```python
from build123d import *

# Parameters (mm, degrees)
SKETCH1_R           = 24.5
SKETCH1_R_2         = 2.4999999999999996
SKETCH1_R_3         = 2.499999999999988
SKETCH1_R_4         = 2.5000000000000018
BOSS_EXTRUDE1_DEPTH = 10.530000000000001
SKETCH2_R           = 4
SKETCH2_R_2         = 2.4999999999999996
BOSS_EXTRUDE2_DEPTH = 14.5
SKETCH3_R           = 5
SKETCH3_R_2         = 4
BOSS_EXTRUDE3_DEPTH = 1.5
BOSS_EXTRUDE4_DEPTH = 14.5
FILLET2_R           = 0.5
FILLET5_R           = 1.5
CIRPATTERN1_START   = 10.53
CIRPATTERN1_DEPTH   = 14.5
SKETCH5_R           = 1.5000000000000442
CUT_EXTRUDE1_DEPTH  = 43.74343124745603
SKETCH6_R           = 2.7499999999999947
CUT_EXTRUDE2_DEPTH  = 3
SKETCH7_R           = 4.25
CUT_EXTRUDE3_DEPTH  = 5
CIRPATTERN2_COUNT   = 3
CHAMFER1_SIZE       = 0.5
SKETCH9_R           = 8
CUT_EXTRUDE4_DEPTH  = 38.559952245709795
BOSS_EXTRUDE7_START = -6.530000000000001
SKETCH10_R          = 8
SKETCH10_R_2        = 6.500000000000002
BOSS_EXTRUDE7_DEPTH = 6.530000000000001
CHAMFER2_SIZE       = 0.5
BOSS_EXTRUDE8_START = -1.5
SKETCH11_R          = 26.000000000000007
SKETCH11_R_2        = 24.5
BOSS_EXTRUDE8_DEPTH = 1.5


# Read off the part's stored shape, not the designer's step: CirPattern1
with BuildPart() as part:
    # Sketch1 → Boss-Extrude1 (new body)
    with BuildSketch(Plane.XY):
        Circle(SKETCH1_R)
        with Locations((0, 19.5)):
            Circle(SKETCH1_R_2, mode=Mode.SUBTRACT)
        with Locations((16.887495373796185, -9.750000000000636)):
            Circle(SKETCH1_R_3, mode=Mode.SUBTRACT)
        with Locations((-16.887495373797307, -9.750000000000002)):
            Circle(SKETCH1_R_4, mode=Mode.SUBTRACT)
    extrude(amount=BOSS_EXTRUDE1_DEPTH)

    # Sketch2 → Boss-Extrude2 (add)
    with BuildSketch(Plane.XY.offset(10.530000000000001)):
        with Locations(Location((0, 19.5, 0), (0, 0, 180))):
            Circle(SKETCH2_R)
        with Locations((0, 19.5)):
            Circle(SKETCH2_R_2, mode=Mode.SUBTRACT)
    extrude(amount=BOSS_EXTRUDE2_DEPTH)

    # Sketch3 → Boss-Extrude3 (add)
    with BuildSketch(Plane.XY.offset(10.530000000000001)):
        with Locations(Location((0, 19.5, 0), (0, 0, 90))):
            Circle(SKETCH3_R)
        with Locations(Location((0, 19.5, 0), (0, 0, 180))):
            Circle(SKETCH3_R_2, mode=Mode.SUBTRACT)
    extrude(amount=BOSS_EXTRUDE3_DEPTH)

    # Sketch4 → Boss-Extrude4 (add)
    with BuildSketch(Plane.XY.offset(10.530000000000001)):
        with BuildLine():
            ThreePointArc((-8.496322733983213, 7.75), (-12.968536294458422, 13.01408708204353), (-14.497844667397978, 19.750000000000004))
            ThreePointArc((-14.497844667397978, 19.75), (-21.21762239271878, 12.249999999999943), (-24.352924058441666, 2.6805017820872727))
            ThreePointArc((-24.352924058441673, 2.6805017820872727), (-17.754798167341832, 4.724038339879645), (-10.959858246321023, 3.48303132638066))
            ThreePointArc((-10.959858246321025, 3.483031326380663), (-9.959292143521058, 5.749999999999978), (-8.496322733983213, 7.750000000000001))
        make_face()
    extrude(amount=BOSS_EXTRUDE4_DEPTH)

    # Fillet2
    fillet2_edges = [part.edges().sort_by_distance(p)[0] for p in [
        (-9.2e-16, 14.5, 12.030000000000001),
    ]]
    fillet(fillet2_edges, radius=FILLET2_R)

    # Fillet5
    fillet5_edges = [part.edges().sort_by_distance(p)[0] for p in [
        (-14.49784466739798, 19.75, 17.78),
        (-24.35292405844167, 2.6805017820872727, 17.78),
        (-10.959858246321025, 3.4830313263806616, 17.78),
        (-8.496322733983215, 7.75, 17.78),
    ]]
    fillet(fillet5_edges, radius=FILLET5_R)

    # CirPattern1 outline → CirPattern1 (add)
    with BuildSketch(Plane.XY.offset(CIRPATTERN1_START)):
        with BuildLine():
            ThreePointArc((-1.069906346, -11.450122288), (-2.103251355, -11.738985499), (-2.679275225, -12.644214953))
            ThreePointArc((-2.679275225, -12.644214953), (-4.43366395, -17.176444835), (-7.58708663, -20.874405476))
            ThreePointArc((-7.58708663, -20.874405476), (-8.094453803, -22.326259468), (-7.057038992, -23.461632523))
            ThreePointArc((-7.057038992, -23.461632523), (0, -24.5), (7.057038992, -23.461632523))
            ThreePointArc((7.057038992, -23.461632523), (8.094453803, -22.326259468), (7.58708663, -20.874405476))
            ThreePointArc((7.58708663, -20.874405476), (4.43366395, -17.176444835), (2.679275225, -12.644214953))
            ThreePointArc((2.679275225, -12.644214953), (2.103251355, -11.738985499), (1.069906346, -11.450122288))
            ThreePointArc((1.069906346, -11.450122288), (0, -11.5), (-1.069906346, -11.450122288))
        make_face()
        with BuildLine():
            ThreePointArc((23.846889276, 5.619241219), (21.217622393, 12.25), (16.789850284, 17.842391304))
            ThreePointArc((16.789850284, 17.842391304), (15.28788097, 18.173132357), (14.284222116, 17.0078125))
            ThreePointArc((14.284222116, 17.0078125), (12.658405598, 12.42788803), (9.610573748, 8.642427885))
            ThreePointArc((9.610573748, 8.642427885), (9.11463398, 7.690961853), (9.381143605, 6.651627219))
            ThreePointArc((9.381143605, 6.651627219), (9.959292144, 5.75), (10.451049951, 4.798495069))
            ThreePointArc((10.451049951, 4.798495069), (11.217885334, 4.048023646), (12.289848972, 4.001787068))
            ThreePointArc((12.289848972, 4.001787068), (17.092069548, 4.748556804), (21.871308746, 3.866592976))
            ThreePointArc((21.871308746, 3.866592976), (23.382334773, 4.153127111), (23.846889276, 5.619241219))
        make_face()
    extrude(amount=CIRPATTERN1_DEPTH)

    # CirPattern1 2 outline → CirPattern1 2 (revolve)
    with BuildSketch(Plane(origin=(-16.887495374, -9.75, 0), x_dir=(1, 0, 0), z_dir=(0, -1, 0))):
        with BuildLine():
            Line((4, 25.03), (2.5, 25.03))
            Line((2.5, 25.03), (2.5, 10.53))
            Line((2.5, 10.53), (5, 10.53))
            Line((5, 10.53), (5, 11.53))
            ThreePointArc((5, 11.53), (4.853553391, 11.883553391), (4.5, 12.03))
            Line((4.5, 12.03), (4, 12.03))
            Line((4, 12.03), (4, 25.03))
        make_face()
    revolve(axis=Axis((-16.887495374, -9.75, 0), (0, 0, 1)))

    # CirPattern1 3 outline → CirPattern1 3 (revolve)
    with BuildSketch(Plane(origin=(16.887495374, -9.75, 0), x_dir=(1, 0, 0), z_dir=(0, -1, 0))):
        with BuildLine():
            Line((4, 25.03), (2.5, 25.03))
            Line((2.5, 25.03), (2.5, 10.53))
            Line((2.5, 10.53), (5, 10.53))
            Line((5, 10.53), (5, 11.53))
            ThreePointArc((5, 11.53), (4.853553391, 11.883553391), (4.5, 12.03))
            Line((4.5, 12.03), (4, 12.03))
            Line((4, 12.03), (4, 25.03))
        make_face()
    revolve(axis=Axis((16.887495374, -9.75, 0), (0, 0, 1)))

    # Sketch5 → Cut-Extrude1 (cut, through all)
    with BuildSketch(Plane.XY.offset(25.030000000000005)):
        with Locations((-17.753520777581024, 10.249999999999956)):
            Circle(SKETCH5_R)
    cut_extrude1 = extrude(amount=-CUT_EXTRUDE1_DEPTH, mode=Mode.SUBTRACT)

    # Sketch6 → Cut-Extrude2 (cut)
    with BuildSketch(Plane(origin=(0, 0, 0), x_dir=(-1, 0, 0), z_dir=(0, 0, -1))):
        with Locations((17.753520777581024, 10.249999999999956)):
            Circle(SKETCH6_R)
    cut_extrude2 = extrude(amount=-CUT_EXTRUDE2_DEPTH, mode=Mode.SUBTRACT)

    # Sketch7 → Cut-Extrude3 (cut)
    with BuildSketch(Plane(origin=(0, 0, 0), x_dir=(-1, 0, 0), z_dir=(0, 0, -1))):
        with Locations((0, 19.5)):
            Circle(SKETCH7_R)
    cut_extrude3 = extrude(amount=-CUT_EXTRUDE3_DEPTH, mode=Mode.SUBTRACT)

    # CirPattern2: Cut-Extrude1, Cut-Extrude2, Cut-Extrude3 ×3 about axis
    cirpattern2_axis = Axis((1.3e-16, -8.9e-16, 0), (0, 0, 1))
    add([cut_extrude1.rotate(cirpattern2_axis, i * 360 / CIRPATTERN2_COUNT) for i in range(1, CIRPATTERN2_COUNT)], mode=Mode.SUBTRACT)
    add([cut_extrude2.rotate(cirpattern2_axis, i * 360 / CIRPATTERN2_COUNT) for i in range(1, CIRPATTERN2_COUNT)], mode=Mode.SUBTRACT)
    add([cut_extrude3.rotate(cirpattern2_axis, i * 360 / CIRPATTERN2_COUNT) for i in range(1, CIRPATTERN2_COUNT)], mode=Mode.SUBTRACT)

    # Chamfer1
    chamfer1_edges = [part.edges().sort_by_distance(p)[0] for p in [
        (-24.5, 3e-15, 0),
    ]]
    chamfer(chamfer1_edges, length=CHAMFER1_SIZE)

    # Sketch9 → Cut-Extrude4 (cut, through all)
    with BuildSketch(Plane.XY.offset(10.530000000000001)):
        Circle(SKETCH9_R)
    extrude(amount=-CUT_EXTRUDE4_DEPTH, mode=Mode.SUBTRACT)

    # Sketch10 → Boss-Extrude7 (add)
    with BuildSketch(Plane(origin=(0, 0, 0), x_dir=(-1, 0, 0), z_dir=(0, 0, -1)).offset(BOSS_EXTRUDE7_START)):
        with Locations(Location((0, 0, 0), (0, 0, 180))):
            Circle(SKETCH10_R)
        Circle(SKETCH10_R_2, mode=Mode.SUBTRACT)
    extrude(amount=BOSS_EXTRUDE7_DEPTH)

    # Chamfer2
    chamfer2_edges = [part.edges().sort_by_distance(p)[0] for p in [
        (-8, 9.8e-16, 10.530000000000001),
    ]]
    chamfer(chamfer2_edges, length=CHAMFER2_SIZE)

    # Sketch11 → Boss-Extrude8 (add)
    with BuildSketch(Plane.XY.offset(10.530000000000001).offset(BOSS_EXTRUDE8_START)):
        Circle(SKETCH11_R)
        Circle(SKETCH11_R_2, mode=Mode.SUBTRACT)
    extrude(amount=BOSS_EXTRUDE8_DEPTH)


solid = part.part
```
Check sheet for the modelled part. Datum: model origin and axes. Units: mm. A direction names the side the tool comes from. Round coordinates to 2 decimals unless told otherwise and drop trailing zeros. Order: outer loops, then holes, each group sorted by start corner. A loop starts at its lowest first (then second) coordinate and runs counter-clockwise, first axis right, second up. Notation, with made-up numbers: (-15.75, 20.25) -> (7.25, 20.25) arc R17 ccw to (7.25, 43.25) -> close; hole circle Ø5 at (-14, 71). An arc over 180 degrees is marked (long way). One line per item, written item: value. Start each with the question number.
Q1. Set-up check for faces 4 (the face through (9.952, 5.763, 17.678)), 5 (the face through (-0.22, 14.505, 11.023)), 6 (the face through (16, -7, 5)): record each of +Z, -Z, +X, -X, +Y, -Y from which the full face is reachable in a straight line by a thin tool's end or side.
Q2. Mould release check, pull along X, two halves, no side actions. Record for faces 1 (the face through (13.17, 20.66, 4.71)), 2 (the face through (17, 12, 3)), 3 (the face through (-16.9, -12.4, 25.03)): pulls with the +X half, pulls with the -X half, needs draft (parallel to the pull), parting line crosses it, or undercut.
Q3. Thickness scan on line 1 (Y direction, x = 0, z = 7.65); line 2 (Y direction, x = 16, z = 20.5); line 3 (X direction, y = 10.5, z = 21.5). Record the ranges inside material, lowest first.
Q4. Cross-section at C-C (x = -18.5). Give the number of separate pieces and of enclosed holes in the cut face, and give its area (3 significant figures).
Q5. Cross-section at B-B (z = 4). Record the boundary of the cut face in (x, y), and give its area (3 significant figures).
Q6. Cross-section at A-A (y = 0). Record the boundary of the cut face in (x, z).
Q7. Gauge pin test, flat ends, axial feed: pin 1 Ø6 at (x, z) = (-9.5, 19.5) entering from +Y; pin 2 Ø3 at (x, y) = (-19.5, 18.5) entering from -Z; pin 3 Ø3 at (y, z) = (-13, 9.5) entering from -X; pin 4 Ø3 at (y, z) = (-3.5, 13.5) entering from -X. Record the tip position at first contact, or that the pin passes through.
Completed:
1. face 4: +Z, -Y
1. face 5: +Z
1. face 6: -Z
2. face 1: parting line crosses it
2. face 2: undercut
2. face 3: needs draft
3. line 1: y = -24.5 to -22, -19 to -8, 8 to 17, 22 to 24.5
3. line 2: y = -13.65 to -12.09, -7.41 to -5.85, 4.72 to 18.23
3. line 3: x = -22.14 to -19.23, -16.27 to -11.37, 11.37 to 16.27, 19.23 to 22.14
4. separate pieces: 3
4. enclosed holes: 0
4. area: 430 mm²
5. outline: circle Ø49 at (0, 0); hole circle Ø8.5 at (-16.89, -9.75); hole circle Ø3 at (-17.75, 10.25); hole circle Ø13 at (0, 0); hole circle Ø8.5 at (0, 19.5); hole circle Ø3 at (0, -20.5); hole circle Ø8.5 at (16.89, -9.75); hole circle Ø3 at (17.75, 10.25)
5. area: 1,560 mm²
6. outline: (-26, 9.03) -> (-24.5, 9.03) -> (-24.5, 0.5) -> (-24, 0) -> (-6.5, 0) -> (-6.5, 6.53) -> (-8, 6.53) -> (-8, 10.03) -> (-8.5, 10.53) -> (-26, 10.53) -> close; (6.5, 0) -> (24, 0) -> (24.5, 0.5) -> (24.5, 9.03) -> (26, 9.03) -> (26, 10.53) -> (8.5, 10.53) -> (8, 10.03) -> (8, 6.53) -> (6.5, 6.53) -> close
7. pin 1: stops at y = 12.15
7. pin 2: stops at z = 9.03
7. pin 3: stops at x = -23.32
7. pin 4: passes through
